Autodesk Inventor part; units mm, degrees
ref_plane "Work Plane1" through (0, 20, 0) normal (0, 1, 0) x (-1, 0, 0)
ref_plane "YZ Plane" through (0, 0, 0) normal (1, 0, 0) x (0, 1, 0)
ref_plane "XY Plane" through (0, 0, 0) normal (0, 0, 1) x (1, 0, 0)
sketch "Sketch1" plane through (0, 0, 0) normal (0, 0, 1) x (1, 0, 0)
  line L0 (0, 0) -> (0, 20)
  line L1 (0, 0) -> (20, 0)
  arc A0 (20, 0) -> (0, 20) centre (0, 0) ccw
  line L2 (0, -4.828427) -> (0, 28.970563)
  dimension "d2" = 20
sketch "Sketch1 outline for Revolution1" plane through (0, 0, 0) normal (0, 0, 1) x (1, 0, 0)
  line L0 (0, 0) -> (0, 20)
  arc A0 (0, 20) -> (20, 0) centre (0, 0) cw
  line L1 (20, 0) -> (0, 0)
revolve "Revolution1" add sketch "Sketch1 outline for Revolution1" angle 360 about axis through (0, -10, 0) along (0, 1, 0)
ref_plane "Work Plane1" through (0, 20, 0) normal (0, 1, 0) x (-1, 0, 0)
sketch "Sketch2" plane through (0, 20, 0) normal (0, 1, 0) x (-1, 0, 0)
  point P0 (0, 0)
  point P1 (0, 0)
hole "Hole1" at (0, 20, 0) direction (0, -1, 0) diameter 4.5 end through all counterbore diameter 8 counterbore depth 4
shell "Shell1" thickness 4 removed faces 1 at (13.884144, 0, 1.68584)
sketch "Sketch3" plane through (0, 0, 0) normal (0, -1, 0) x (1, 0, 0)
  circle A0 centre (0, 0) radius 2.25
  circle A1 centre (0, 0) radius 6.25
  circle A2 centre (0, 0) radius 2.25
sketch "Sketch3 outline for Extrusion1" plane through (0, 0, 0) normal (0, -1, 0) x (1, 0, 0)
  circle A0 centre (0, 0) radius 6.25
  circle A1 centre (0, 0) radius 2.25
extrude "Extrusion1" cut sketch "Sketch3 outline for Extrusion1" against normal up to surface (12 mm away)
properties part number "Ball_Upper Half" material "Nylon 6/6"
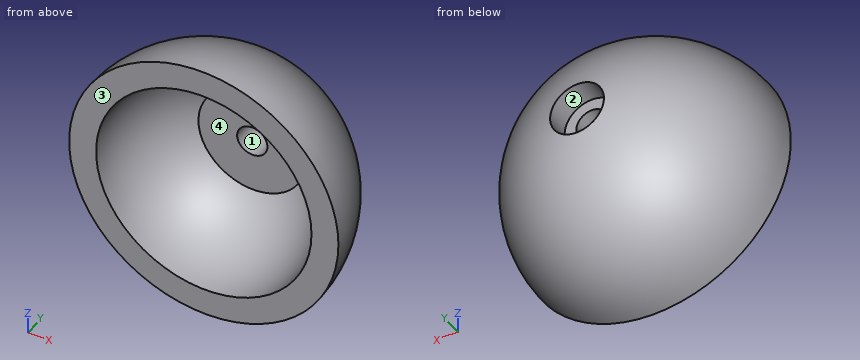
The listing builds one solid part. Answer for the finished solid, in the listing's coordinates (mm). Face numbers are marked on the shaded views. A direction names the side the tool comes from. Coordinates: 2 decimals unless noted, no trailing zeros. Write each loop counter-clockwise with the first axis right and the second up, starting at its lowest first coordinate (ties: lowest second). Pieces come first, ordered by that corner, then holes. Notation, with made-up numbers: (77.5, 88.5) - (108.5, 88.5) arc R21 ccw to (108.5, 107.5) - close; hole circle Ø7 at (-12.75, -28.5). An arc over 180 degrees is marked (long way). Return JSON: item names as keys, results as strings. Group by question number.
Q1. Flat-ended cylindrical pins translate along their axes: pin 1 Ø6 at (x, z) = (0, 0) entering from -Y; pin 2 Ø4 at (y, z) = (10, 2.5) entering from -X; pin 3 Ø2.5 at (x, z) = (1.5, 1.5) entering from +Y; pin 4 Ø6 at (x, z) = (1.5, 0) entering from +Y. Find the tip coordinate at first contact, or state that the pin passes through.
Q2. Which of the six approach directions +Z, -Z, +X, -X, +Y, -Y give full straight-line access (tool end or side, diameter ignored) to the marked faces 1 and 2?
Q3. The part is cut by section C-C on x = -6. Write down the section's boundary in (y, z), and give its area (3 significant figures).
Q4. The part is cut by section A-A on z = 0. Write down the section's boundary in (x, y).
Q5. The part is cut by section D-D on z = -7.5. Write down the section's boundary in (x, y).
Q6. The part is cut by section B-B on y = 13.25. Write down the section's boundary in (x, z), and give its area (3 significant figures).
Q7. Find the intervals of material crossed by line 1 along X through (y, z) = (13.45, 0); line 2 along X through (y, z) = (17.05, 0); line 3 along X through (y, z) = (14, 0), in increasing order. Write a range as [from, to].
Q8. For a pull along X with two mould halves and no side action, classify the marked faces 3 and 4 as +X half, -X half, draft (parallel to the pull), parting line (faces both ways), or undercut.
Evaluation:
{
 "1": {"pin 1": "stops at y = 12", "pin 2": "stops at x = -18.19", "pin 3": "stops at y = 16", "pin 4": "stops at y = 19.6"},
 "2": {"face 1": "+Y, -Y", "face 2": "+Y"},
 "3": {"outline": "(0, -19.08) arc R19.08 ccw to (0, 19.08) - (0, 14.83) arc R14.83 cw to (13.86, 5.29) - (12, 5.29) - (12, -5.29) - (13.86, -5.29) arc R14.83 cw to (0, -14.83) - close", "area": "253 mm2"},
 "4": {"outline": "(-20, 0) - (-16, 0) arc R16 cw to (-8, 13.86) - (-8, 12) - (-2.25, 12) - (-2.25, 16) - (-4, 16) - (-4, 19.6) arc R20 ccw to start; (2.25, 12) - (8, 12) - (8, 13.86) arc R16 cw to (16, 0) - (20, 0) arc R20 ccw to (4, 19.6) - (4, 16) - (2.25, 16) - close"},
 "5": {"outline": "(-18.54, 0) - (-14.13, 0) arc R14.13 cw to (-2.78, 13.86) - (-2.78, 12) - (2.78, 12) - (2.78, 13.86) arc R14.13 cw to (14.13, 0) - (18.54, 0) arc R18.54 ccw to start"},
 "6": {"outline": "circle Ø29.96 at (0, 0); circle Ø16 at (0, 0); hole circle Ø17.94 at (0, 0); hole circle Ø4.5 at (0, 0)", "area": "638 mm2"},
 "7": {"line 1": "x = [-14.8, -8.67], [-8, -2.25], [2.25, 8], [8.67, 14.8]", "line 2": "x = [-10.45, -4], [4, 10.45]", "line 3": "x = [-14.28, -2.25], [2.25, 14.28]"},
 "8": {"face 3": "draft", "face 4": "undercut"}
}
